```python
from build123d import *

# Parameters (mm, degrees)
SKETCH_3_R          = 1.6
CUT_EXTRUDE_1_DEPTH = 64.287719075


with BuildPart() as part:
    # ｽｹｯﾁ2 → 回転1 (revolve)
    with BuildSketch(Plane(origin=(0, 0, 0), x_dir=(1, 0, 0), z_dir=(0, 1, 0)), mode=Mode.PRIVATE) as revolve_1_sk:
        Polygon((-44.73085458, -0.056036178), (-44.73085458, -17.056036178), (-30.73085458, -17.056036178), (-30.73085458, -0.056036178), (-31.73085458, -0.056036178), (-31.73085458, -5.056036178), (-43.73085458, -5.056036178), (-43.73085458, -0.056036178), align=None)
    revolve(revolve_1_sk.sketch.rotate(Axis((-49.849406884, 0, 20.056036178), (1, 0, 0)), 180), axis=Axis((-49.849406884, 0, 20.056036178), (1, 0, 0)))

    # ｽｹｯﾁ3 → ｶｯﾄ - 押し出し1 (cut, through all)
    with BuildSketch(Plane(origin=(0, 0, 0), x_dir=(1, 0, 0), z_dir=(0, 1, 0))):
        with Locations(Location((-37.73085458, -20.056036178, 0), (0, 0, 270))):
            Circle(SKETCH_3_R)
    extrude(amount=-CUT_EXTRUDE_1_DEPTH, mode=Mode.SUBTRACT)


solid = part.part
```
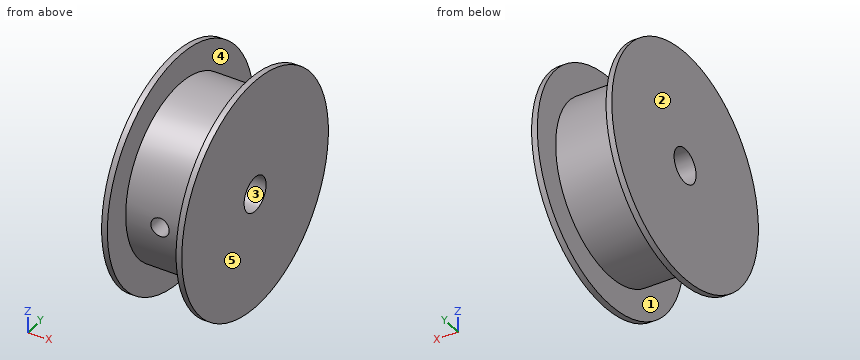
Could you check a few things on this model? Use its own coordinates, in mm. Face numbers are marked on the shaded views. A direction names the side the tool comes from. Give positions to 0.01 mm unless a question says otherwise; leave off trailing zeros. Write each loop counter-clockwise with the first axis right and the second up, starting at its lowest first coordinate (ties: lowest second). Pieces come first, ordered by that corner, then holes. Notation, with made-up numbers: (6.25, 30) - (52.25, 30) arc R8 cw to (52.25, 41) - close; hole circle Ø6 at (55.5, 71). An arc over 180 degrees is marked (long way). One line per item, written item: value. Start each with the question number.
Item 1: Imagine slicing it at B-B, the plane z = 3. List the corners of the cut face in (x, y) for me.
Item 2: Imagine slicing it at C-C, the plane x = -40. List the corners of the cut face in (y, z) for me, and give its area (3 significant figures).
Item 3: Imagine slicing it at D-D, the plane z = 13. List the corners of the cut face in (x, y) for me.
Item 4: I'm going to push flat-ended pins straight in: pin 1 (3 mm diameter, centred on x = -40.5, y = 0, fed in from -Z); pin 2 (3.5 mm diameter, centred on x = -37.73, z = 20.06, fed in from +Y); pin 3 (5 mm diameter, centred on x = -43, z = 34.5, fed in from -Y). Where does each tip first touch, or does it pass through?
Item 5: Imagine slicing it at A-A, the plane y = 0. List the corners of the cut face in (x, z) for me.
Item 6: Please list where these lines run through material, in increasing order: line 1 (X direction, y = 18, z = 27.5); line 2 (X direction, y = -7, z = 19); line 3 (Z direction, x = -38.5, y = 7.5). Write a range as from..to.
Item 7: Which directions (+Z, -Z, +X, -X, +Y, -Y) give clear straight access to the entire face, cutting with the end or side of a thin tool? Please do the marked faces 1 and 2.
Item 8: If we mould it in two halves opening along X, with no side actions, what happens to the marked faces 3, 4 and 5? For each: +X half, -X half, draft (parallel to the pull), parting line (faces both ways), or undercut.
Geometry says:
1. outline: (-44.73, -10.44) - (-43.73, -10.44) - (-43.73, 10.44) - (-44.73, 10.44) - close; (-31.73, -10.44) - (-30.73, -10.44) - (-30.73, 10.44) - (-31.73, 10.44) - close
2. outline: circle Ø30 at (0, 20.06); hole circle Ø6 at (0, 20.06)
2. area: 679 mm^2
3. outline: (-44.73, -18.71) - (-43.73, -18.71) - (-43.73, -13.24) - (-31.73, -13.24) - (-31.73, -18.71) - (-30.73, -18.71) - (-30.73, 18.71) - (-31.73, 18.71) - (-31.73, 13.24) - (-43.73, 13.24) - (-43.73, 18.71) - (-44.73, 18.71) - close
4. pin 1: z = 5.06
4. pin 2: y = 15
4. pin 3: y = -15.96
5. outline: (-44.73, 0.06) - (-43.73, 0.06) - (-43.73, 5.06) - (-31.73, 5.06) - (-31.73, 0.06) - (-30.73, 0.06) - (-30.73, 17.06) - (-44.73, 17.06) - close; (-44.73, 23.06) - (-30.73, 23.06) - (-30.73, 40.06) - (-31.73, 40.06) - (-31.73, 35.06) - (-43.73, 35.06) - (-43.73, 40.06) - (-44.73, 40.06) - close
6. line 1: -44.73..-43.73, -31.73..-30.73
6. line 2: -44.73..-38.93, -36.53..-30.73
6. line 3: 7.07..33.05
7. face 1: none
7. face 2: +Z, -Z, -X, +Y, -Y
8. face 3: draft
8. face 4: undercut
8. face 5: +X half
